Verification items for the finished model (mm, model axes). A direction names the side the tool comes from. Give positions to 0.01 mm unless a question says otherwise; leave off trailing zeros. Write each loop counter-clockwise with the first axis right and the second up, starting at its lowest first coordinate (ties: lowest second). Pieces come first, ordered by that corner, then holes. Notation, with made-up numbers: (-10, 1.25) -> (26, 1.25) arc R19 cw to (26, 16.25) -> close; hole circle Ø8 at (-20.75, -10.75). An arc over 180 degrees is marked (long way). Answer as CSV lines item,"result".
Autodesk Inventor part; units mm, degrees
ref_plane "YZ Plane" through (0, 0, 0) normal (1, 0, 0) x (0, 1, 0)
ref_plane "XZ Plane" through (0, 0, 0) normal (0, 1, 0) x (-1, 0, 0)
ref_plane "XY Plane" through (0, 0, 0) normal (0, 0, 1) x (1, 0, 0)
sketch "Sketch2" plane through (0, 0, 0) normal (0, 0, 1) x (1, 0, 0)
  circle A0 centre (4.5, -2.75) radius 1.25
  line L0 (9.5, 7.5) -> (-5, 7.5)
  line L1 (-5, 7.5) -> (-5, 2)
  line L2 (-5, 2) -> (-0.5, 2)
  line L3 (-0.5, 2) -> (-0.5, -7.5)
  line L4 (-0.5, -7.5) -> (7.5, -7.5)
  line L5 (9.5, -5.5) -> (9.5, 7.5)
  circle A1 centre (4.75, -38) radius 1.25
  line L6 (-5, -45.5) -> (8, -45.5)
  line L7 (10, -43.5) -> (10, -32.5)
  line L8 (8, -30.5) -> (-0.5, -30.5)
  line L9 (-0.5, -30.5) -> (-0.5, -40)
  line L10 (-0.5, -40) -> (-5, -40)
  line L11 (-5, -40) -> (-5, -45.5)
  circle A2 centre (-47.5, -38) radius 1.25
  line L12 (-38, -40) -> (-42.5, -40)
  line L13 (-42.5, -40) -> (-42.5, -30.5)
  line L14 (-42.5, -30.5) -> (-50.5, -30.5)
  line L15 (-52.5, -32.5) -> (-52.5, -43.5)
  line L16 (-50.5, -45.5) -> (-38, -45.5)
  line L17 (-38, -45.5) -> (-38, -40)
  circle A3 centre (-47.5, 0) radius 1.25
  line L18 (-42.5, -7.5) -> (-42.5, 2)
  line L19 (-42.5, 2) -> (-38, 2)
  line L20 (-38, 2) -> (-38, 7.5)
  line L21 (-38, 7.5) -> (-50.5, 7.5)
  line L22 (-52.5, 5.5) -> (-52.5, -5.5)
  line L23 (-50.5, -7.5) -> (-42.5, -7.5)
  circle A4 centre (-21.1548, -18.9993) radius 2.5
  circle A5 centre (-21.1548, -18.9993) radius 12.5
  line L24 (-0.5, 2) -> (-42.5, 2)
  line L25 (-42.5, 2) -> (-42.5, -40)
  line L26 (-42.5, -40) -> (-0.5, -40)
  line L27 (-0.5, -40) -> (-0.5, 2)
  arc A6 (-52.5, -5.5) -> (-50.5, -7.5) centre (-50.5, -5.5) ccw
  arc A7 (-50.5, 7.5) -> (-52.5, 5.5) centre (-50.5, 5.5) ccw
  arc A8 (8, -45.5) -> (10, -43.5) centre (8, -43.5) ccw
  arc A9 (10, -32.5) -> (8, -30.5) centre (8, -32.5) ccw
  arc A10 (7.5, -7.5) -> (9.5, -5.5) centre (7.5, -5.5) ccw
  arc A11 (-52.5, -43.5) -> (-50.5, -45.5) centre (-50.5, -43.5) ccw
  arc A12 (-50.5, -30.5) -> (-52.5, -32.5) centre (-50.5, -32.5) ccw
  line L28 (9.5, 2) -> (-52.5, 2)
  line L29 (9.5, 2) -> (-52.5, 2)
  point P0 (0, 0)
extrude "Extrusion1" add sketch "Sketch2" along normal blind 5 contours L5 L28 L2 L1 L0 | L5 A10 L4 L3 L28 | L2 L3 L27 L9 L10 L26 L12 L13 L25 L18 L19 L24 | L19 L28 L22 A7 L21 L20 | L18 L23 A6 L22 L28 | L8 A9 L7 A8 L6 L11 L10 L9 | L13 L12 L17 L16 A11 L15 A12 L14
properties part number "Drzalo_motorja"
1) Depth check by flat-ended pin: pin 1 (1 mm diameter, centred on x = -28, z = 3, fed in from +Y); pin 2 (22.5 mm diameter, centred on x = -21.15, y = -19, fed in from -Z); pin 3 (1.5 mm diameter, centred on y = 3.5, z = 2.5, fed in from +X). Enter the tip coordinate at first touch or a pass-through.
Reported:
pin 1,"y = 2"
pin 2,"through"
pin 3,"x = 9.5"
2) Draft check along X on faces 1 (the cylindrical face through (-48.49, -37.24, 2.46)), 2 (the cylindrical face through (-51.93, 6.9, 2.46)), 3 (the cylindrical face through (4.34, -3.99, 2.46)), 4 (the flat face through (-0.5, -19, 2)). Enter one of: +X half, -X half, draft (parallel to the pull), parting line (faces both ways), or undercut.
Reported:
face 1,"undercut"
face 2,"-X half"
face 3,"undercut"
face 4,"+X half"
3) Scan lines: line 1 along X through (y, z) = (-3.5, 2.4); line 2 along Y through (x, z) = (2, 3.7); line 3 along X through (y, z) = (-19.5, 3.3). Record each from-to range of solid material in increasing order.
Reported:
line 1,"-52.5 to 3.5, 5.5 to 9.5"
line 2,"-45.5 to -30.5, -7.5 to 7.5"
line 3,"-42.5 to -33.64, -8.66 to -0.5"
4) Section check A-A (y = -38). Record the boundary of the cut face in (x, z), and give its area (4 significant figures).
Reported:
outline,"(-52.5, 0) -> (-48.75, 0) -> (-48.75, 5) -> (-52.5, 5) -> close; (-46.25, 0) -> (3.5, 0) -> (3.5, 5) -> (-46.25, 5) -> close; (6, 0) -> (10, 0) -> (10, 5) -> (6, 5) -> close"
area,"287.5 mm²"
5) Tool access check on faces 5 (the flat face through (-38, -43, 2)), 6 (the flat face through (-42.5, -19, 2)), 7 (the flat face through (-38, 5, 2)), 8 (the cylindrical face through (8.93, -6.9, 2.46)). Record the directions out of +Z, -Z, +X, -X, +Y, -Y that give a thin tool (end or side, any length) a straight path to the whole face; none if there is none.
Reported:
face 5,"+Z, -Z, -Y"
face 6,"+Z, -Z, -X"
face 7,"+Z, -Z, +Y"
face 8,"+Z, -Z, +X"
6) Section check B-B (x = -11.5). Record the boundary of the cut face in (y, z).
Reported:
outline,"(-40, 0) -> (-26.94, 0) -> (-26.94, 5) -> (-40, 5) -> close; (-11.06, 0) -> (2, 0) -> (2, 5) -> (-11.06, 5) -> close"
7) Section check C-C (y = -2.75). Record the boundary of the cut face in (x, z).
Reported:
outline,"(-52.5, 0) -> (3.25, 0) -> (3.25, 5) -> (-52.5, 5) -> close; (5.75, 0) -> (9.5, 0) -> (9.5, 5) -> (5.75, 5) -> close"
8) Section check D-D (x = -47.5). Record the boundary of the cut face in (y, z).
Reported:
outline,"(-45.5, 0) -> (-39.25, 0) -> (-39.25, 5) -> (-45.5, 5) -> close; (-36.75, 0) -> (-30.5, 0) -> (-30.5, 5) -> (-36.75, 5) -> close; (-7.5, 0) -> (-1.25, 0) -> (-1.25, 5) -> (-7.5, 5) -> close; (1.25, 0) -> (7.5, 0) -> (7.5, 5) -> (1.25, 5) -> close"
